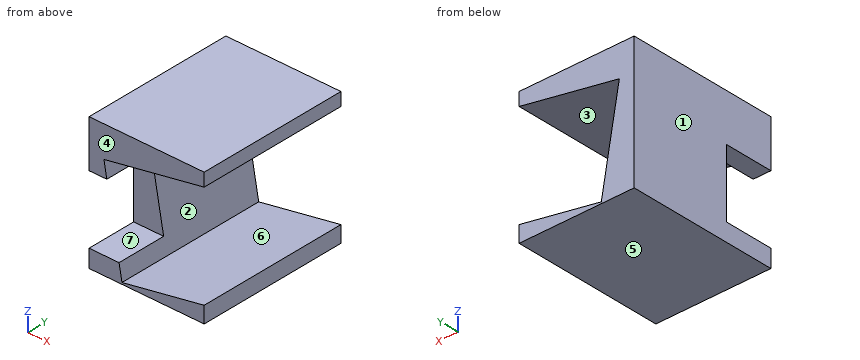
```python
from build123d import *

# Parameters (mm, degrees)
BASE_DEPTH = 18.4


with BuildPart() as part:
    # Croquis17 → BASE (new body)
    with BuildSketch(Plane(origin=(0, 0, 0), x_dir=(-1, 0, 0), z_dir=(0, 1, 0))):
        Polygon((0, 0), (-10, 1.8), (-10, -0.2), (4, -0.2), (4, 15.99927871), (-10, 15.99927871), (-10, 14.39927871), (2.196697179, 12.203873217), align=None)
    extrude(amount=-BASE_DEPTH)

    # Croquis19 → WIRE_WINDOW section 0
    with BuildSketch(Plane(origin=(0, 0, 0), x_dir=(0, 1, 0), z_dir=(0.9841833239736953, 0, 0.17715299831526504))):
        with BuildLine():
            Line((-18.4, 10.4), (-12.4, 10.4))
            Line((-12.4, 10.4), (-12.4, 2))
            Line((-12.4, 2), (-18.4, 2))
            Line((-18.4, 2), (-18.4, 10.4))
        make_face()
    # Croquis20 → WIRE_WINDOW section 1
    with BuildSketch(Plane(origin=(-4, 0, 0), x_dir=(0, -1, 0), z_dir=(-1, 0, 0))):
        with BuildLine():
            Line((18.4, 1.968366648), (12.4, 1.968366648))
            Line((12.4, 1.968366648), (12.4, 10.235506569))
            Line((12.4, 10.235506569), (18.4, 10.235506569))
            Line((18.4, 10.235506569), (18.4, 1.968366648))
        make_face()
    loft(mode=Mode.SUBTRACT)


solid = part.part
```
CAD build for the part. Positions are in the model's coordinates, mm. Face numbers are marked on the shaded views. A direction names the side the tool comes from. Round coordinates to 2 decimals unless told otherwise and drop trailing zeros. Loops run counter-clockwise (first coordinate to the right, second up) from the corner with the lowest first, then second, coordinate; pieces in that order, holes last. Notation, with made-up numbers: M 24,48.25 L 63,48.25 A34 cw 63,80.25 Z; hole C 35,48.25 d4. An arc over 180 degrees is marked long. Use a Markdown table: item, result. Add a question column.
(1) Pull direction X, two halves, no side cores. Call the marked faces 1, 2, 3 and 4: +X half, -X half, draft (parallel to the pull), parting line (faces both ways), or undercut.
(2) Cut at D-D (z = 11.5). Give the cut face in (x, y), and give its area (3 significant figures).
(3) Cut at C-C (y = -1.5). Give the cut face in (x, z).
(4) Flat gauge pins, fed straight in: pin 1 (1.5 mm diameter, centred on x = -1.5, z = 7.5, fed in from -Y); pin 2 (2 mm diameter, centred on y = -2, z = 5.5, fed in from +X). Where does each tip first touch, or does it go through?
(5) Cut at A-A (y = -16.5). Give the cut face in (x, z).
(6) Cut at B-B (x = 8.75). Give the cut face in (y, z) (3 decimals), and give its area (3 significant figures).
(7) Which spindle directions (+Z, -Z, +X, -X, +Y, -Y) get a long thin tool onto all of the face, cutting with end or side? Do the marked faces 5, 6 and 7. Say none if no direction does.
(8) Drill centre lines: line 1 (Z direction, x = 3, y = -16); line 2 (Z direction, x = 1.5, y = -6); line 3 (X direction, y = -12, z = 6.5). Where is each one in solid material? Low to high.
Geometry says:
| question | item | result |
|---|---|---|
| 1 | face 1 | -X half |
| 1 | face 2 | undercut |
| 1 | face 3 | +X half |
| 1 | face 4 | draft |
| 2 | outline | M -4,-18.4 L -2.07,-18.4 L -2.07,0 L -4,0 Z |
| 2 | area | 35.5 mm² |
| 3 | outline | M -4,-0.2 L 10,-0.2 L 10,1.8 L 0,0 L -2.2,12.2 L 10,14.4 L 10,16 L -4,16 Z |
| 4 | pin 1 | stops at y = -12.4 |
| 4 | pin 2 | stops at x = -0.81 |
| 5 | outline | M -4,-0.2 L 10,-0.2 L 10,1.8 L 0,0 L -0.35,1.97 L -4,1.97 Z; M -4,10.24 L -1.84,10.24 L -2.2,12.2 L 10,14.4 L 10,16 L -4,16 Z |
| 6 | outline | M -18.4,-0.2 L 0,-0.2 L 0,1.575 L -18.4,1.575 Z; M -18.4,14.174 L 0,14.174 L 0,15.999 L -18.4,15.999 Z |
| 6 | area | 66.2 mm² |
| 7 | face 5 | -Z, +X, -X, +Y, -Y |
| 7 | face 6 | +Y, -Y |
| 7 | face 7 | +X, -X, -Y |
| 8 | line 1 | z = -0.2 to 0.54, 13.14 to 16 |
| 8 | line 2 | z = -0.2 to 0.27, 12.87 to 16 |
| 8 | line 3 | x = -4 to -1.17 |
